The listing builds one solid part. Answer for the finished solid, in the listing's coordinates (mm). Face numbers are marked on the shaded views. A direction names the side the tool comes from. Round coordinates to 2 decimals unless told otherwise and drop trailing zeros. Write each loop counter-clockwise with the first axis right and the second up, starting at its lowest first coordinate (ties: lowest second). Pieces come first, ordered by that corner, then holes.
Item 1: Find section A-A on z = 0. Give the vertices of the cut face in (x, y), then the cut area to 3 significant figures.
Item 2: For a pull along X with two mould halves and no side action, classify the marked faces 4, 5 and 6 as +X half, -X half, draft (parallel to the pull), parting line (faces both ways), or undercut.
Item 3: Find section C-C on x = 22.5. Give the vertices of the cut face in (y, z), then the cut area to 3 significant figures.
Item 4: A tool of negligible diameter and unlimited length cuts with its end or side. For the marked faces 1, 2 and 3, from which of +Z, -Z, +X, -X, +Y, -Y can it reach the whole face along a straight path? Write none if from no direction.
Item 5: Each of these flat-tipped pins is pushed along its axis until it touches: pin 1 (2 mm diameter, centred on y = -13.1, z = 17.29, fed in from +X); pin 2 (3 mm diameter, centred on x = 13.5, z = 44.5, fed in from -Y); pin 3 (5 mm diameter, centred on x = 19.5, y = -13, fed in from -Z); pin 4 (4 mm diameter, centred on x = 4, z = 43.5, fed in from +Y). Where does it stop, or does it pass through?
Item 6: Find section B-B on y = 51.42. Give the vertices of the cut face in (x, z), then the cut area to 3 significant figures.
Item 7: Find section D-D on y = 6.5. Give the vertices of the cut face in (x, z), then the cut area to 3 significant figures.
Item 8: Find the intervals of material crossed by probe 1 along Y at (x, z) = (1.3, 0); probe 2 along Z at (x, y) = (4.5, 3); probe 3 along Y at (x, z) = (20.35, -16.22), in increasing order.
```python
from build123d import *

# Parameters (mm, degrees)
SKETCH1_W                                       = 15
SKETCH1_H                                       = 45
BOSS_EXTRUDE1_DEPTH                             = 5
SKETCH2_W                                       = 15
SKETCH2_H                                       = 15
BOSS_EXTRUDE2_DEPTH                             = 14
SKETCH3_R                                       = 2.3
CUT_EXTRUDE1_DEPTH                              = 7
SKETCH4_R                                       = 7.5
SKETCH4_R_2                                     = 1.65
BOSS_EXTRUDE3_DEPTH                             = 6
CSK_FOR_M3_FLAT_HEAD_MACHINE_SCREW1_D           = 3.4
CSK_FOR_M3_FLAT_HEAD_MACHINE_SCREW1_DEPTH       = 6.35
CSK_FOR_M3_FLAT_HEAD_MACHINE_SCREW1_CSINK_D     = 6.3
CSK_FOR_M3_FLAT_HEAD_MACHINE_SCREW1_CSINK_ANGLE = 90
CSK_FOR_M3_FLAT_HEAD_MACHINE_SCREW1_TIP         = 1.021463052


with BuildPart() as part:
    # Sketch1 → Boss-Extrude1 (new body)
    with BuildSketch(Plane(origin=(0, 0, 0), x_dir=(0, 0, -1), z_dir=(1, 0, 0))):
        with BuildLine():
            Line((-33.857008974, 2.735870452), (-45.565370995, -7.267550065))
            ThreePointArc((-45.565370995, -7.267550065), (-27.604171468, -17.561381798), (-7.5, -22.5))
            Line((-7.5, -22.5), (-7.5, -7.403306871))
            ThreePointArc((-7.5, -7.403306871), (-21.290873092, -3.925583536), (-33.857008974, 2.735870452))
        make_face()
        Rectangle(SKETCH1_W, SKETCH1_H)
        with BuildLine():
            Line((-41.931432124, 9.489065709), (-52.538033842, -1.117536008))
            ThreePointArc((-52.538033842, -1.117536008), (-49.147992618, -4.301713372), (-45.565370995, -7.267550065))
            Line((-45.565370995, -7.267550065), (-33.857008974, 2.735870452))
            ThreePointArc((-33.857008974, 2.735870452), (-38.044360457, 5.932954073), (-41.931432124, 9.489065709))
        make_face()
    extrude(amount=BOSS_EXTRUDE1_DEPTH)

    # Sketch2 → Boss-Extrude2 (add)
    with BuildSketch(Plane(origin=(5, 0, 0), x_dir=(0, 0, -1), z_dir=(1, 0, 0))):
        with BuildLine():
            Line((-45.563203072, -7.269233174), (-33.854727787, 2.734284113))
            ThreePointArc((-33.854727787, 2.734284113), (-29.354954434, -0.104026911), (-24.61890521, -2.52762082))
            Line((-24.61890521, -2.52762082), (-36.933994133, -13.049418231))
            ThreePointArc((-36.933994133, -13.049418231), (-41.349722145, -10.310292527), (-45.563203072, -7.269233174))
        make_face()
        with Locations((0, 15)):
            Rectangle(SKETCH2_W, SKETCH2_H)
    extrude(amount=BOSS_EXTRUDE2_DEPTH)

    # Sketch3 → Cut-Extrude1 (cut)
    with BuildSketch(Plane(origin=(5, 0, 0), x_dir=(0, 0, -1), z_dir=(1, 0, 0))):
        with Locations((-39.70896543, -2.267474531)):
            Circle(SKETCH3_R)
    extrude(amount=CUT_EXTRUDE1_DEPTH, mode=Mode.SUBTRACT)

    # Sketch4 → Boss-Extrude3 (add)
    with BuildSketch(Plane(origin=(19, 0, 0), x_dir=(0, 0, -1), z_dir=(1, 0, 0))):
        with BuildLine():
            Line((-7.5, 33.697965455), (-7.5, 7.5))
            Line((-7.5, 7.5), (7.5, 7.5))
            Line((7.5, 7.5), (7.5, 33.697965455))
            Line((7.5, 33.697965455), (9.165031814, 33.697965455))
            ThreePointArc((9.165031814, 33.697965455), (9.933965272, 34.117264651), (10.683756157, 34.569905907))
            Line((10.683756157, 34.569905907), (13.30556247, 36.552911383))
            ThreePointArc((13.30556247, 36.552911383), (13.786023096, 36.997313573), (14.25164947, 37.457235089))
            Line((14.25164947, 37.457235089), (14.25164947, 45.3641606))
            Line((14.25164947, 45.3641606), (24.03628358, 48.30778647))
            ThreePointArc((24.03628358, 48.30778647), (26.349985315, 51.429769983), (24.017555191, 54.53778647))
            Line((24.017555191, 54.53778647), (14.241296463, 57.414910041))
            ThreePointArc((14.241296463, 57.414910041), (0, 66.87164947), (-14.241296463, 57.414910041))
            Line((-14.241296463, 57.414910041), (-24.017555191, 54.53778647))
            ThreePointArc((-24.017555191, 54.53778647), (-26.349985315, 51.429769983), (-24.03628358, 48.30778647))
            Line((-24.03628358, 48.30778647), (-14.25164947, 45.3641606))
            Line((-14.25164947, 45.3641606), (-14.25164947, 37.457235089))
            ThreePointArc((-14.25164947, 37.457235089), (-13.786023096, 36.997313573), (-13.30556247, 36.552911383))
            Line((-13.30556247, 36.552911383), (-10.683756157, 34.569905907))
            ThreePointArc((-10.683756157, 34.569905907), (-9.933965272, 34.117264651), (-9.165031814, 33.697965455))
            Line((-9.165031814, 33.697965455), (-7.5, 33.697965455))
        make_face()
        with Locations((0, 51.42)):
            Circle(SKETCH4_R, mode=Mode.SUBTRACT)
        with Locations((16.22, 51.42)):
            Circle(SKETCH4_R_2, mode=Mode.SUBTRACT)
        with Locations((-16.22, 51.42)):
            Circle(SKETCH4_R_2, mode=Mode.SUBTRACT)
    extrude(amount=BOSS_EXTRUDE3_DEPTH)

    # CSK for M3 Flat Head Machine Screw1
    with Locations(Plane(origin=(5, 0, 0), x_dir=(0, 0, -1), z_dir=(1, 0, 0))):
        with Locations((-42.74343682, 0.09035829), (-17.288987754, -13.103380711), (0, 0), (0, 51.42)):
            CounterSinkHole(CSK_FOR_M3_FLAT_HEAD_MACHINE_SCREW1_D / 2, CSK_FOR_M3_FLAT_HEAD_MACHINE_SCREW1_CSINK_D / 2, depth=CSK_FOR_M3_FLAT_HEAD_MACHINE_SCREW1_DEPTH, counter_sink_angle=CSK_FOR_M3_FLAT_HEAD_MACHINE_SCREW1_CSINK_ANGLE)
            with Locations((0, 0, -(CSK_FOR_M3_FLAT_HEAD_MACHINE_SCREW1_DEPTH + CSK_FOR_M3_FLAT_HEAD_MACHINE_SCREW1_TIP / 2))):  # 118° drill point
                Cone(0, CSK_FOR_M3_FLAT_HEAD_MACHINE_SCREW1_D / 2, CSK_FOR_M3_FLAT_HEAD_MACHINE_SCREW1_TIP, mode=Mode.SUBTRACT)


solid = part.part
```
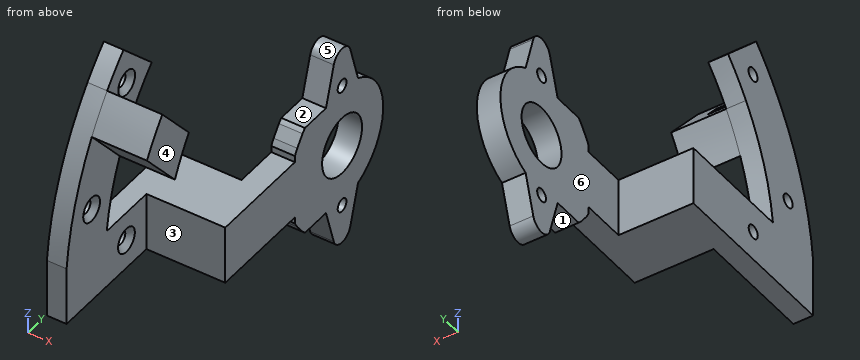
Check values:
1. outline: (0, -22.5) - (5, -22.5) - (5, -3.15) - (3.55, -1.7) - (0, -1.7) - close; (0, 1.7) - (3.55, 1.7) - (5, 3.15) - (5, 7.5) - (25, 7.5) - (25, 43.92) - (19, 43.92) - (19, 22.5) - (0, 22.5) - close; (19, 58.92) - (25, 58.92) - (25, 66.87) - (19, 66.87) - close
1. area: 682 mm2
2. face 4: +X half
2. face 5: draft
2. face 6: -X half
3. outline: (7.5, -7.5) - (33.7, -7.5) - (33.7, -9.17) arc R19.95 ccw to (34.57, -10.68) - (36.55, -13.31) arc R19.95 ccw to (37.46, -14.25) - (45.36, -14.25) - (48.31, -24.04) arc R3.25 ccw to (54.54, -24.02) - (57.41, -14.24) arc R15.45 ccw to (57.41, 14.24) - (54.54, 24.02) arc R3.25 ccw to (48.31, 24.04) - (45.36, 14.25) - (37.46, 14.25) arc R19.95 ccw to (36.55, 13.31) - (34.57, 10.68) arc R19.95 ccw to (33.7, 9.17) - (33.7, 7.5) - (7.5, 7.5) - close; hole circle Ø15 at (51.42, 0); hole circle Ø3.3 at (51.42, -16.22); hole circle Ø3.3 at (51.42, 16.22)
3. area: 1,250 mm2
4. face 1: -Z, +X, -X, -Y
4. face 2: +Z, +X, -X, -Y
4. face 3: +Z, -Z, +X, -Y
5. pin 1: passes through
5. pin 2: stops at y = -9.17
5. pin 3: stops at z = 34.01
5. pin 4: stops at y = 9.49
6. outline: (19, -26.35) - (25, -26.35) - (25, -17.87) - (19, -17.87) - close; (19, -14.57) - (25, -14.57) - (25, -7.5) - (19, -7.5) - close; (19, 7.5) - (25, 7.5) - (25, 14.57) - (19, 14.57) - close; (19, 17.87) - (25, 17.87) - (25, 26.35) - (19, 26.35) - close
6. area: 187 mm2
7. outline: (0, -7.5) - (5, -7.5) - (5, 7.5) - (0, 7.5) - close; (0, 38.71) - (5, 38.71) - (5, 44.92) - (0, 44.92) - close
7. area: 106 mm2
8. probe 1: y = -22.5 to -1.7, 1.7 to 22.5
8. probe 2: z = -7.5 to 7.5, 34.23 to 48.42
8. probe 3: y = 45.96 to 49.77, 53.07 to 56.83
